Check sheet for the drawn part. Datum: minimum x, y, z corner. Units: mm. A direction names the side the tool comes from. Coordinates: 2 decimals unless noted, no trailing zeros. Loops run counter-clockwise (first coordinate to the right, second up) from the corner with the lowest first, then second, coordinate; pieces in that order, holes last. Notation, with made-up numbers: (-4.75, -8.75) -> (51.25, -8.75) arc R22 ccw to (51.25, 6.25) -> close; hole circle Ø1 at (14.5, 70). An arc over 180 degrees is marked (long way). Use CSV: the item, a comma, the result in double quotes. Start each with the question number.
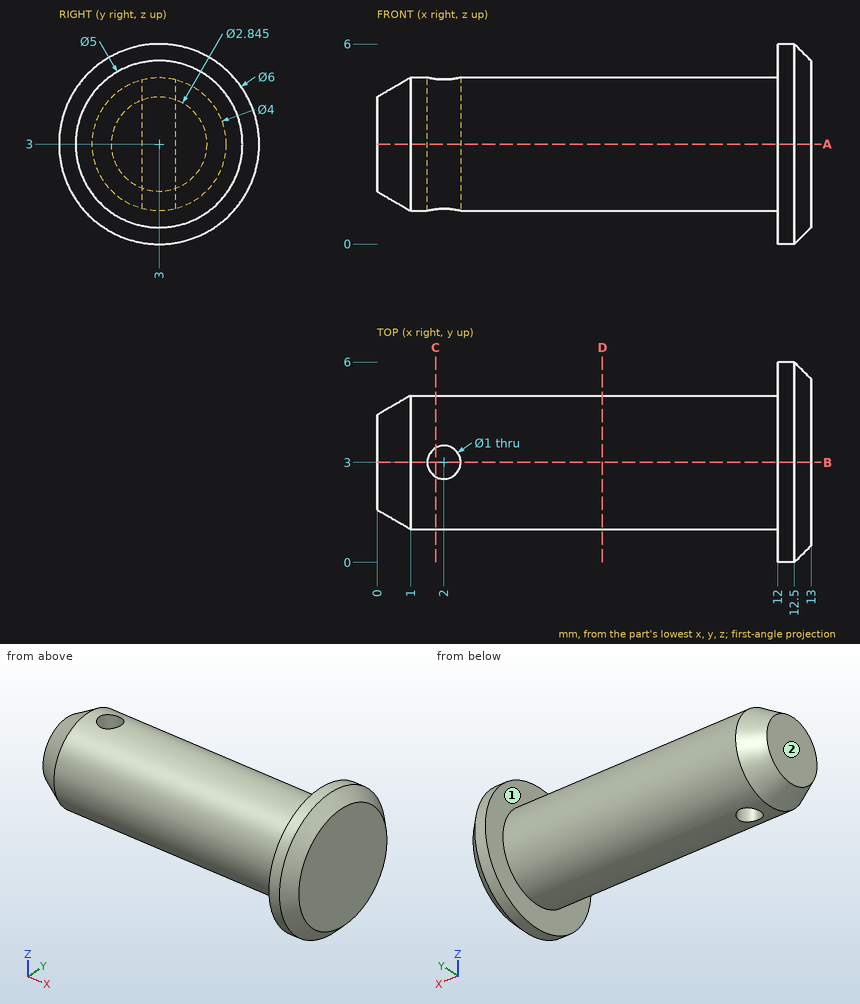
1. Cross-section at C-C, the plane x = 1.75. Record the boundary of the cut face in (y, z).
2. Cross-section at D-D, the plane x = 6.75. Record the boundary of the cut face in (y, z).
3. Cross-section at A-A, the plane z = 3. Record the boundary of the cut face in (x, y).
4. Cross-section at B-B, the plane y = 3. Record the boundary of the cut face in (x, z).
5. Scan lines: line 1 (X direction, y = 3, z = 4); line 2 (Y direction, x = 2, z = 2.95); line 3 (Z direction, x = 5, y = 2.9). Record each from-to range of solid material in increasing order.
6. Depth check by flat-ended pin: pin 1 (1.5 mm diameter, centred on x = 2, z = 4.5, fed in from -Y); pin 2 (1.5 mm diameter, centred on x = 9, z = 5, fed in from +Y); pin 3 (1 mm diameter, centred on y = 1, z = 2, fed in from -X). Enter the tip coordinate at first touch or a pass-through.
7. Set-up check for the marked faces 1 and 2: record each of +Z, -Z, +X, -X, +Y, -Y from which the full face is reachable in a straight line by a thin tool's end or side.
Solution:
1,outline,"(2.57, 1.05) -> (2.57, 4.95) arc R2 ccw to start; (3.43, 1.05) arc R2 ccw to (3.43, 4.95) -> close"
2,outline,"circle Ø4 at (3, 3)"
3,outline,"(0, 1.58) -> (1, 1) -> (12, 1) -> (12, 0) -> (12.5, 0) -> (13, 0.5) -> (13, 5.5) -> (12.5, 6) -> (12, 6) -> (12, 5) -> (1, 5) -> (0, 4.42) -> close; hole circle Ø1 at (2, 3)"
4,outline,"(0, 1.58) -> (1, 1) -> (1.5, 1) -> (1.5, 5) -> (1, 5) -> (0, 4.42) -> close; (2.5, 1) -> (12, 1) -> (12, 0) -> (12.5, 0) -> (13, 0.5) -> (13, 5.5) -> (12.5, 6) -> (12, 6) -> (12, 5) -> (2.5, 5) -> close"
5,line 1,"x = 0 to 1.5, 2.5 to 13"
5,line 2,"y = 1 to 2.5, 3.5 to 5"
5,line 3,"z = 1 to 5"
6,pin 1,"stops at y = 1.15"
6,pin 2,"stops at y = 4.56"
6,pin 3,"stops at x = 0.54"
7,face 1,"-X"
7,face 2,"+Z, -Z, -X, +Y, -Y"
